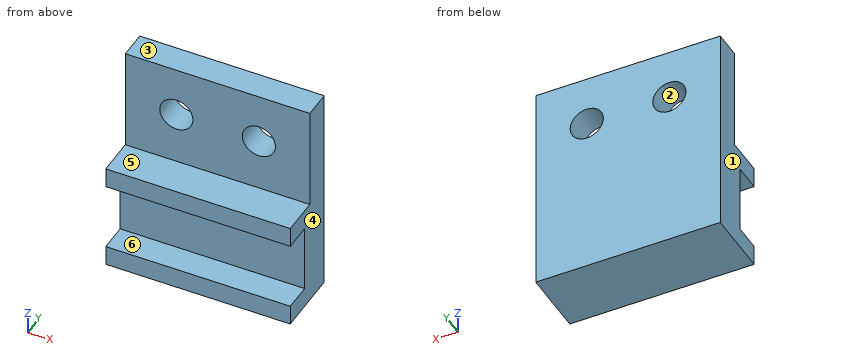
from build123d import *

# Parameters (mm, degrees)
F0_W     = 114.935
F0_H     = 65.0875
F0_R     = 10.31875
F0_H_2   = 12.7
F0_H_3   = 42.8625
F1_DEPTH = 17.4625
F2_DEPTH = 23.8125
F3_DEPTH = 41.275


with BuildPart() as f1:
    # F0 (on Front) → F1 (new body)
    with BuildSketch(Plane.XZ):
        with Locations((-10.257453, 33.324088)):
            Rectangle(F0_W, F0_H)
        with Locations((-35.972588, 34.117838)):
            Circle(F0_R, mode=Mode.SUBTRACT)
        with Locations((15.460047, 34.117838)):
            Circle(F0_R, mode=Mode.SUBTRACT)
        with Locations((-10.257453, -5.569662)):
            Rectangle(F0_W, F0_H_2)
        with Locations((-10.257453, -33.350912)):
            Rectangle(F0_W, F0_H_3)
        with Locations((-10.257453, -61.132162)):
            Rectangle(F0_W, F0_H_2)
    extrude(amount=F1_DEPTH)

    # F0 (on Front) → F2 (join)
    with BuildSketch(Plane.XZ):
        with Locations((-10.257453, -61.132162)):
            Rectangle(F0_W, F0_H_2)
        with Locations((-10.257453, -33.350912)):
            Rectangle(F0_W, F0_H_3)
        with Locations((-10.257453, -5.569662)):
            Rectangle(F0_W, F0_H_2)
    extrude(amount=F2_DEPTH)

    # F0 (on Front) → F3 (join)
    with BuildSketch(Plane.XZ):
        with Locations((-10.257453, -5.569662)):
            Rectangle(F0_W, F0_H_2)
        with Locations((-10.257453, -61.132162)):
            Rectangle(F0_W, F0_H_2)
    extrude(amount=F3_DEPTH)


solid = f1.part
Build history of the part. All positions in model axes, mm. Face numbers are marked on the shaded views. A direction names the side the tool comes from. Round coordinates to 2 decimals unless told otherwise and drop trailing zeros. Write each loop counter-clockwise with the first axis right and the second up, starting at its lowest first coordinate (ties: lowest second). Pieces come first, ordered by that corner, then holes. Notation, with made-up numbers: M 47,74.5 L 92,74.5 A17 ccw 92,104.5 Z; hole C 15,-35 d8. An arc over 180 degrees is marked long. Use CSV: the item, a comma, the result in double quotes.
1. Saw through at D-D (x = -4). Give the cut face in (y, z) (1 decimal), plus the area to 3 significant figures.
Reply:
outline,"M -41.3,-67.5 L 0,-67.5 L 0,65.9 L -17.5,65.9 L -17.5,0.8 L -41.3,0.8 L -41.3,-11.9 L -23.8,-11.9 L -23.8,-54.8 L -41.3,-54.8 Z"
area,"3,210 mm²"
2. Two-plate mould, pull along Z, no slides. Class the marked faces 1, 2 and 3: +Z half, -Z half, draft (parallel to the pull), parting line (faces both ways), or undercut.
Reply:
face 1,"draft"
face 2,"undercut"
face 3,"+Z half"
3. Saw through at A-A (y = -37). Give the cut face in (x, z), plus the area to 3 significant figures.
Reply:
outline,"M -67.72,-67.48 L 47.21,-67.48 L 47.21,-54.78 L -67.72,-54.78 Z; M -67.72,-11.92 L 47.21,-11.92 L 47.21,0.78 L -67.72,0.78 Z"
area,"2,920 mm²"
4. Saw through at B-B (z = 41.5). Give the cut face in (x, y), plus the area to 3 significant figures.
Reply:
outline,"M -67.72,-17.46 L -43.18,-17.46 L -43.18,0 L -67.72,0 Z; M -28.76,-17.46 L 8.25,-17.46 L 8.25,0 L -28.76,0 Z; M 22.67,-17.46 L 47.21,-17.46 L 47.21,0 L 22.67,0 Z"
area,"1,500 mm²"
5. Tool access for the marked faces 4, 5 and 6: list every direction of +Z, -Z, +X, -X, +Y, -Y with a clear straight run to the whole face (end or side of a thin tool).
Reply:
face 4,"+Z, -Z, +X, +Y, -Y"
face 5,"+Z, +X, -X, -Y"
face 6,"+X, -X, -Y"
6. Saw through at C-C (x = -27.5). Give the cut face in (y, z) (1 decimal), plus the area to 3 significant figures.
Reply:
outline,"M -41.3,-67.5 L 0,-67.5 L 0,28.2 L -17.5,28.2 L -17.5,0.8 L -41.3,0.8 L -41.3,-11.9 L -23.8,-11.9 L -23.8,-54.8 L -41.3,-54.8 Z; M -17.5,40 L 0,40 L 0,65.9 L -17.5,65.9 Z"
area,"3,000 mm²"
7. Wall check: probe 1 along Z at (x, y) = (-59, -33); probe 2 along Y at (x, z) = (12, 51.5); probe 3 along Z at (x, y) = (-6, -23). Give the ranges that are in metal, low to high. Write a range as from..to.
Reply:
probe 1,"z = -67.48..-54.78, -11.92..0.78"
probe 2,"y = -17.46..0"
probe 3,"z = -67.48..0.78"
8. Flat gauge pins, fed straight in: pin 1 (8.5 mm diameter, centred on x = -7, y = -36, fed in from +Z); pin 2 (16.5 mm diameter, centred on x = 15.46, z = 34.12, fed in from -Y); pin 3 (4 mm diameter, centred on x = -40, z = -14, fed in from -Y); pin 4 (19.5 mm diameter, centred on x = -30.5, z = 29, fed in from -Y). Where does each tip first touch, or does it go through?
Reply:
pin 1,"stops at z = 0.78"
pin 2,"passes through"
pin 3,"stops at y = -23.81"
pin 4,"stops at y = -17.46"
